Source: three-view drawing plus pictorial views. Frame: mm from the lowest corner of the part. A direction names the side the tool comes from. Give positions to 0.01 mm unless a question says otherwise; leave off trailing zeros. Order: outer loops, then holes, each group sorted by start corner. A loop starts at its lowest first (then second) coordinate and runs counter-clockwise, first axis right, second up. Notation, with made-up numbers: (78, 34.5) - (119, 34.5) arc R27 ccw to (119, 55.5) - close; hole circle Ø10 at (-24, 55). An arc over 180 degrees is marked (long way). Use CSV: the item, a comma, the result in double quotes.
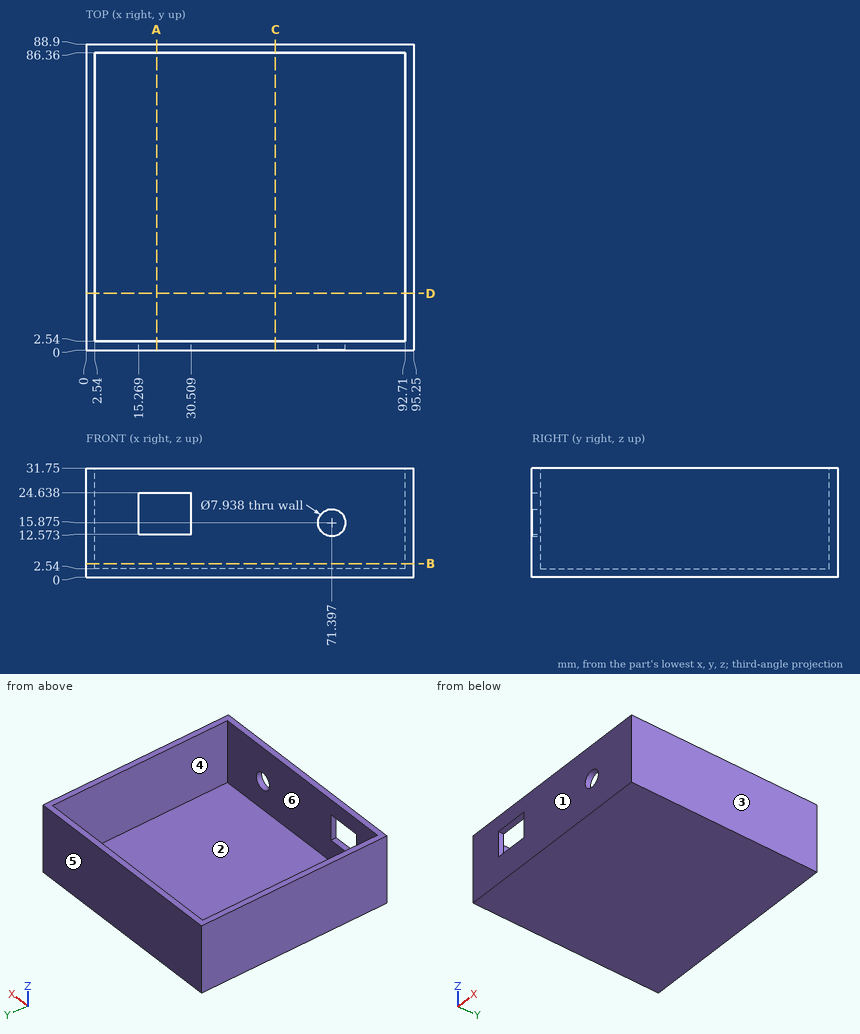
Item 1: Material intervals for line 1 (Y direction, x = 13.5, z = 10); line 2 (X direction, y = 16, z = 16); line 3 (Z direction, x = 59.5, y = 78), sorted ascending. Write a range as from..to.
Filled in:
line 1,"y = 0..2.54, 86.36..88.9"
line 2,"x = 0..2.54, 92.71..95.25"
line 3,"z = 0..2.54"
Item 2: Section B-B on z = 4. Return the cut outline in (x, y).
Filled in:
outline,"(0, 0) - (95.25, 0) - (95.25, 88.9) - (0, 88.9) - close; hole (2.54, 2.54) - (92.71, 2.54) - (92.71, 86.36) - (2.54, 86.36) - close"
Item 3: First-contact query: pin 1 (3 mm diameter, centred on x = 69, y = 9.5, fed in from +Z). Flat tip, straight axial feed; report the tip coordinate or a pass-through.
Filled in:
pin 1,"stops at z = 2.54"
Item 4: Section D-D on y = 16.5. Return the cut outline in (x, z).
Filled in:
outline,"(0, 0) - (95.25, 0) - (95.25, 31.75) - (92.71, 31.75) - (92.71, 2.54) - (2.54, 2.54) - (2.54, 31.75) - (0, 31.75) - close"
Item 5: Mould query, pull axis Y, two halves, no side actions, for the marked faces 1, 2, 3 and 4. Classes: released by +Y, released by -Y, zero draft, split by the parting line, or undercut.
Filled in:
face 1,"released by -Y"
face 2,"undercut"
face 3,"zero draft"
face 4,"undercut"
Item 6: Set-up query: the marked faces 5 and 6. Return all of +Z, -Z, +X, -X, +Y, -Y with unobstructed straight access to the full face (end or side cutting, diameter ignored); none if empty.
Filled in:
face 5,"+Z, -Z, +X, -X, +Y"
face 6,"+Z"
Item 7: Section C-C on x = 55. Return the cut outline in (y, z), then the cut area to 3 significant figures.
Filled in:
outline,"(0, 0) - (88.9, 0) - (88.9, 31.75) - (86.36, 31.75) - (86.36, 2.54) - (2.54, 2.54) - (2.54, 31.75) - (0, 31.75) - close"
area,"374 mm2"
Item 8: Section A-A on x = 20.5. Return the cut outline in (y, z).
Filled in:
outline,"(0, 0) - (88.9, 0) - (88.9, 31.75) - (86.36, 31.75) - (86.36, 2.54) - (2.54, 2.54) - (2.54, 12.57) - (0, 12.57) - close; (0, 24.64) - (2.54, 24.64) - (2.54, 31.75) - (0, 31.75) - close"
